Answer from the drawing. Dimensions are ordinates in mm from the lowest x, y and z of the part. Give positions to 0.01 mm unless a question says otherwise; leave off trailing zeros. Write each loop counter-clockwise with the first axis right and the second up, starting at its lowest first coordinate (ties: lowest second). Pieces come first, ordered by that corner, then holes.
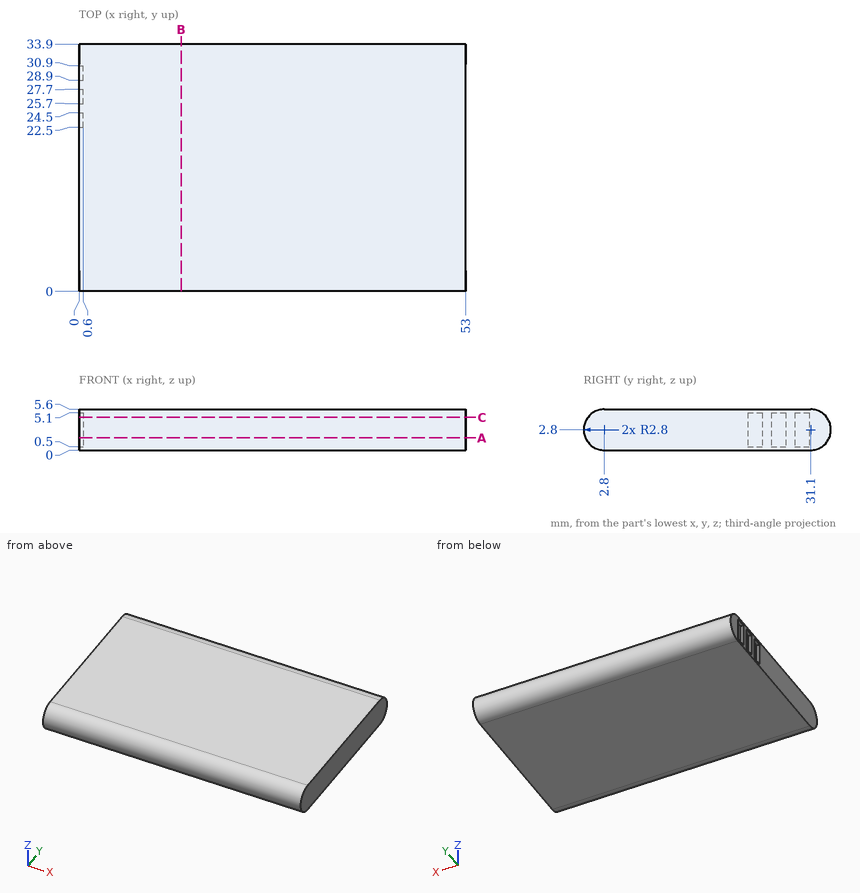
Item 1: A cutting plane is placed at C-C, the plane z = 4.5. Give the vertices of the cut face in (x, y), plus the area to 3 significant figures.
Conclusion:
outline: (0, 0.58) - (53, 0.58) - (53, 33.32) - (0, 33.32) - (0, 30.9) - (0.6, 30.9) - (0.6, 28.9) - (0, 28.9) - (0, 27.7) - (0.6, 27.7) - (0.6, 25.7) - (0, 25.7) - (0, 24.5) - (0.6, 24.5) - (0.6, 22.5) - (0, 22.5) - close
area: 1,730 mm2
Item 2: A cutting plane is placed at B-B, the plane x = 14. Give the vertices of the cut face in (y, z), plus the area to 3 significant figures.
Conclusion:
outline: (2.8, 0) - (31.1, 0) arc R2.8 ccw to (31.1, 5.6) - (2.8, 5.6) arc R2.8 ccw to start
area: 183 mm2
Item 3: A cutting plane is placed at A-A, the plane z = 1.7. Give the vertices of the cut face in (x, y).
Conclusion:
outline: (0, 0.23) - (53, 0.23) - (53, 33.67) - (0, 33.67) - (0, 30.9) - (0.6, 30.9) - (0.6, 28.9) - (0, 28.9) - (0, 27.7) - (0.6, 27.7) - (0.6, 25.7) - (0, 25.7) - (0, 24.5) - (0.6, 24.5) - (0.6, 22.5) - (0, 22.5) - close
Item 4: Each of these flat-tipped pins is pushed along its axis until it touches: P1, Ø1, axis at x = 43.5, z = 3, coming from the -Y side; P2, Ø1, axis at y = 26.5, z = 3, coming from the -X side. Where does it stop, or does it pass through?
Conclusion:
P1: stops at y = 0
P2: stops at x = 0.6
Item 5: Consider probe 1 along Y at (x, z) = (40, 3); probe 2 along X at (y, z) = (30.5, 4.4); probe 3 along Y at (x, z) = (33, 2). Determine where each line is inside the solid, lowest interval first.
Conclusion:
probe 1: y = 0.01 to 33.89
probe 2: x = 0.6 to 53
probe 3: y = 0.12 to 33.78
